Geometry check sheet. Reference: the model listing, model coordinates, mm. A direction names the side the tool comes from. Coordinates: 2 decimals unless noted, no trailing zeros. Write each loop counter-clockwise with the first axis right and the second up, starting at its lowest first coordinate (ties: lowest second). Pieces come first, ordered by that corner, then holes.
from build123d import *

# Parameters (mm, degrees)
SKETCH1_R                = 3.175
BOSS_EXTRUDE1_DEPTH      = 38.1
BOSS_EXTRUDE2_DEPTH      = 6.35
FILLET1_R                = 3.175
BOSS_EXTRUDE3_DEPTH      = 3.81
BOSS_EXTRUDE3_DEPTH_BACK = 10.16
SKETCH3_W                = 12.7
SKETCH3_H                = 63.5
FILLET2_R                = 3.175
FILLET3_R                = 6.35
CUT_EXTRUDE1_REACH       = 94.13
SKETCH4_W                = 15.24
SKETCH4_H                = 7.62
SKETCH5_R                = 3.175
BOSS_EXTRUDE4_DEPTH      = 10.16


with BuildPart() as part:
    # Sketch1 → Boss-Extrude1 (new body)
    with BuildSketch(Plane(origin=(0, 0, 0), x_dir=(1, 0, 0), z_dir=(0, 1, 0))):
        with Locations(Location((0, 0, 0), (0, 0, 270))):
            Circle(SKETCH1_R)
    extrude(amount=-BOSS_EXTRUDE1_DEPTH)

    # Sketch2 → Boss-Extrude2 (add)
    with BuildSketch(Plane(origin=(0, 0, 0), x_dir=(1, 0, 0), z_dir=(0, 1, 0))):
        Polygon((34.925, -3.175), (-3.175, -3.175), (-3.175, 3.175), (28.575, 3.175), (28.575, 60.325), (34.925, 60.325), align=None)
    extrude(amount=BOSS_EXTRUDE2_DEPTH)

    # Fillet1
    fillet1_edges = [part.edges().sort_by_distance(p)[0] for p in [
        (28.575, 3.175, -3.175),
        (34.925, 3.175, 3.175),
        (-3.175, 3.175, -3.175),
        (-3.175, 3.175, 3.175),
    ]]
    fillet(fillet1_edges, radius=FILLET1_R - 0.0001)  # a hair under: the kernel refuses the full size

    # Sketch3 → Boss-Extrude3 (add, two sides: drawn at the far end of the back side and taken through both)
    with BuildSketch(Plane(origin=(0, 6.35, 0), x_dir=(1, 0, 0), z_dir=(0, 1, 0)).offset(-BOSS_EXTRUDE3_DEPTH_BACK)):
        with Locations((31.75, 41.275)):
            Rectangle(SKETCH3_W, SKETCH3_H)
    extrude(amount=BOSS_EXTRUDE3_DEPTH + BOSS_EXTRUDE3_DEPTH_BACK)

    # Fillet2
    fillet2_edges = [part.edges().sort_by_distance(p)[0] for p in [
        (28.575, 3.175, -9.525),
        (31.75, 0, -9.525),
        (34.925, 3.175, -9.525),
        (31.75, 6.35, -9.525),
    ]]
    fillet(fillet2_edges, radius=FILLET2_R - 0.0001)  # a hair under: the kernel refuses the full size

    # Fillet3
    fillet3_edges = [part.edges().sort_by_distance(p)[0] for p in [
        (25.4, 3.175, -73.025),
        (38.1, 3.175, -73.025),
    ]]
    fillet(fillet3_edges, radius=FILLET3_R - 0.0001)  # a hair under: the kernel refuses the full size

    # Sketch4 → Cut-Extrude1 (cut, up to next)
    with BuildSketch(Plane(origin=(38.1, 0, 0), x_dir=(0, 0, -1), z_dir=(1, 0, 0)), mode=Mode.PRIVATE) as cut_extrude1_sk1:
        with Locations((66.675, 3.175)):
            Rectangle(SKETCH4_W, SKETCH4_H)
    cut_extrude1_tool1 = extrude(cut_extrude1_sk1.sketch, amount=-CUT_EXTRUDE1_REACH, mode=Mode.PRIVATE) & part.part
    add(cut_extrude1_tool1.solids().sort_by_distance((38.1, 3.175, -66.675))[0], mode=Mode.SUBTRACT)

    # Sketch5 → Boss-Extrude4 (add)
    with BuildSketch(Plane(origin=(0, -0.635, 0), x_dir=(1, 0, 0), z_dir=(0, 1, 0))):
        with Locations(Location((31.75, 66.675, 0), (0, 0, 90))):
            Circle(SKETCH5_R)
    extrude(amount=BOSS_EXTRUDE4_DEPTH)


solid = part.part
1. Draft check along Z on faces 4 (the cylindrical face through (31.84, 7.73, -8.97)), 5 (the flat face through (13, 3, -3.175)), 6 (the cylindrical face through (27.62, 3.22, -4.08)). Enter one of: released by +Z, released by -Z, zero draft, split by the parting line, or undercut.
Computed values:
face 4: released by +Z
face 5: released by -Z
face 6: undercut
2. Gauge pin test, flat ends, axial feed: pin 1 Ø1.5 at (x, y) = (1, -3) entering from -Z; pin 2 Ø11 at (y, z) = (3, -50.5) entering from -X; pin 3 Ø10 at (x, z) = (31, -65.5) entering from -Y; pin 4 Ø1.6 at (x, z) = (-2.5, 2) entering from -Y. Record the tip position at first contact, or that the pin passes through.
Computed values:
pin 1: stops at z = -3.17
pin 2: stops at x = 25.4
pin 3: stops at y = -3.81
pin 4: stops at y = -38.1
3. Sectioned sample at B-B, the plane y = -8. Record the boundary of the cut face in (x, z) (3 decimals), and give its area (3 significant figures).
Computed values:
outline: circle Ø6.35 at (0, 0)
area: 31.7 mm2
4. Sectioned sample at C-C, the plane z = -13.5. Record the boundary of the cut face in (x, y), and give its area (3 significant figures).
Computed values:
outline: (25.4, -3.81) - (38.1, -3.81) - (38.1, 10.16) - (25.4, 10.16) - close
area: 177 mm2
5. Sectioned sample at D-D, the plane x = 13. Record the boundary of the cut face in (y, z) (3 decimals), and give its area (3 significant figures).
Computed values:
outline: (0, -3.175) - (6.35, -3.175) - (6.35, 3.175) - (0, 3.175) - close
area: 40.3 mm2
6. Access from +Z, -Z, +X, -X, +Y, -Y to the whole of each face (thin tool, end or side, straight path). Record for faces 1 (the flat face through (32, 6.985, -63)), 2 (the cylindrical face through (27.19, 3.09, -8.97)), 3 (the cylindrical face through (-1.93, -18.78, -2.52)).
Computed values:
face 1: none
face 2: -X, +Y, -Y
face 3: -Y
7. Thickness scan on line 1 along Z through (x, y) = (26.5, 6) (3 decimals); line 2 along X through (y, z) = (7, -52); line 3 along Y through (x, z) = (29.5, -4.5). Record the ranges inside material, lowest first.
Computed values:
line 1: z = -59.055 to -9.328, -3.372 to 3.175
line 2: x = 25.4 to 38.1
line 3: y = 0 to 6.35
8. Sectioned sample at A-A, the plane x = 26.5. Record the boundary of the cut face in (y, z) (3 decimals), and give its area (3 significant figures).
Computed values:
outline: (-3.81, -70.247) - (-0.635, -70.247) - (-0.635, -59.055) - (6.985, -59.055) - (6.985, -70.247) - (10.16, -70.247) - (10.16, -9.525) - (9.525, -9.525) arc R3.175 cw to (8.425, -9.328) - (-2.075, -9.328) arc R3.175 cw to (-3.175, -9.525) - (-3.81, -9.525) - close; (0, -3.372) - (6.35, -3.372) - (6.35, 3.175) - (0, 3.175) - close
area: 807 mm2
